Source: CAD feature listing. Evaluate the final solid. Frame: model axes, mm. A direction names the side the tool comes from. Give positions to 0.01 mm unless a question says otherwise; leave off trailing zeros. Order: outer loops, then holes, each group sorted by start corner. A loop starts at its lowest first (then second) coordinate and runs counter-clockwise, first axis right, second up.
```python
from build123d import *

# Parameters (mm, degrees)
SKETCH1_W           = 200
SKETCH1_H           = 200
BOSS_EXTRUDE2_DEPTH = 100
BOSS_EXTRUDE3_DEPTH = 10
CUT_EXTRUDE1_DEPTH  = 10
SKETCH4_W           = 120
SKETCH4_H           = 20
SKETCH4_W_2         = 20
SKETCH4_H_2         = 120
CUT_EXTRUDE2_DEPTH  = 229.910462845
SKETCH5_R           = 5
CUT_EXTRUDE3_DEPTH  = 314.687742827
SKETCH6_R           = 5
CUT_EXTRUDE4_DEPTH  = 288.054001888
SKETCH7_W           = 103.597474358
SKETCH7_H           = 100
CUT_EXTRUDE7_DEPTH  = 281.178514522
FILLET1_R           = 20


with BuildPart() as part:
    # Sketch1 → Boss-Extrude2 (new body)
    with BuildSketch(Plane(origin=(0, 0, 0), x_dir=(1, 0, 0), z_dir=(0, 1, 0))):
        Rectangle(SKETCH1_W, SKETCH1_H)
    extrude(amount=BOSS_EXTRUDE2_DEPTH)

    # Sketch2 → Boss-Extrude3 (add)
    with BuildSketch(Plane.ZY.offset(-100)):
        with BuildLine():
            Line((140, 10), (-140, 10))
            ThreePointArc((-140, 10), (-180, 50), (-140, 90))
            Line((-140, 90), (140, 90))
            ThreePointArc((140, 90), (180, 50), (140, 10))
        make_face()
    extrude(amount=BOSS_EXTRUDE3_DEPTH)

    # Sketch3 → Cut-Extrude1 (cut)
    with BuildSketch(Plane(origin=(0, 100, 0), x_dir=(1, 0, 0), z_dir=(0, 1, 0))):
        Polygon((8, 25), (8, 50), (94.602540378, 0), (8, -50), (8, -25), (-92, -25), (-92, 25), align=None)
    extrude(amount=-CUT_EXTRUDE1_DEPTH, mode=Mode.SUBTRACT)

    # Sketch4 → Cut-Extrude2 (cut, through all)
    with BuildSketch(Plane(origin=(0, 100, 0), x_dir=(1, 0, 0), z_dir=(0, 1, 0))):
        with Locations((20, 0)):
            Rectangle(SKETCH4_W, SKETCH4_H)
        with Locations((-70, 0)):
            Rectangle(SKETCH4_W_2, SKETCH4_H_2)
    extrude(amount=-CUT_EXTRUDE2_DEPTH, mode=Mode.SUBTRACT)

    # Sketch5 → Cut-Extrude3 (cut, through all)
    with BuildSketch(Plane.XY.offset(100)):
        with Locations((20.147207668, 50)):
            Circle(SKETCH5_R)
    extrude(amount=-CUT_EXTRUDE3_DEPTH, mode=Mode.SUBTRACT)

    # Sketch6 → Cut-Extrude4 (cut, through all)
    with BuildSketch(Plane.ZY.offset(100)):
        with Locations((0, 50)):
            Circle(SKETCH6_R)
    extrude(amount=-CUT_EXTRUDE4_DEPTH, mode=Mode.SUBTRACT)

    # Sketch7 → Cut-Extrude7 (cut, through all)
    with BuildSketch(Plane.ZY.offset(-90)):
        with Locations((-128.201262821, 50)):
            Rectangle(SKETCH7_W, SKETCH7_H)
        with Locations((128.201262821, 50)):
            Rectangle(SKETCH7_W, SKETCH7_H)
    extrude(amount=CUT_EXTRUDE7_DEPTH, mode=Mode.SUBTRACT)

    # Fillet1
    # the kernel refuses this fillet: 20 mm, written as the material it adds along each edge
    with BuildSketch(Plane(origin=(100, 10, -100), x_dir=(0, -1, 0), z_dir=(-1, 0, 0)), Plane(origin=(90, 10, 100), x_dir=(0, -1, 0), z_dir=(1, 0, 0))) as fillet1_piece_1:
        with BuildLine():
            CenterArc((20, -17.320508076), FILLET1_R, 120, 60)
            Line((0, -17.320508076), (-0.4, -17.320508076))
            Line((-0.4, -17.320508076), (-0.4, 0))
            Line((-0.4, 0), (0, 0.4))
            ThreePointArc((0, 0.4), (5, 0.4), (9.8, 0.346410162))
            Line((9.8, 0.346410162), (10, 0))
        make_face()
    extrude(amount=10)
    with BuildSketch(Plane(origin=(90, 90, -100), x_dir=(0, 0, -1), z_dir=(1, 0, 0)), Plane(origin=(100, 90, 100), x_dir=(0, 0, 1), z_dir=(-1, 0, 0))) as fillet1_piece_2:
        with BuildLine():
            CenterArc((17.320508076, 20), FILLET1_R, 210, 60)
            Line((0, 10), (-0.346410162, 9.8))
            ThreePointArc((-0.346410162, 9.8), (-0.4, 5), (-0.4, 0))
            Line((-0.4, 0), (0, -0.4))
            Line((0, -0.4), (17.320508076, -0.4))
            Line((17.320508076, -0.4), (17.320508076, 0))
        make_face()
    extrude(amount=10)


solid = part.part
```
1) Section query B-B, the plane x = 3. Return the cut outline in (y, z).
Report:
outline: (0, -76.4) - (100, -76.4) - (100, -25) - (90, -25) - (90, -10) - (0, -10) - close; (0, 10) - (90, 10) - (90, 25) - (100, 25) - (100, 76.4) - (0, 76.4) - close
2) Material intervals for L1, parallel to X at y = 36.5, z = 7; L2, parallel to Z at x = -90.5, y = 94.5; L3, parallel to Y at x = 95, z = 0, sorted ascending.
Report:
L1: x = -100 to -80, -60 to -40, 80 to 100
L2: z = -76.4 to -25, 25 to 76.4
L3: y = 0 to 45, 55 to 100
3) Section query A-A, the plane z = -56. Return the cut outline in (x, y), and give its area (3 significant figures).
Report:
outline: (-100, 0) - (-80, 0) - (-80, 100) - (-100, 100) - close; (-60, 0) - (100, 0) - (100, 100) - (-60, 100) - close; hole circle Ø10 at (20.15, 50)
area: 17,900 mm2
4) Reachability of faces 4 (the flat face through (95, 90, -129)), 5 (the flat face through (19, 40, -10)), 6 (the flat face through (-26, 95, 25)) from +Z, -Z, +X, -X, +Y, -Y: full face, straight path, thin tool, end or side. Return the list, or none.
Report:
face 4: -Z, +X, -X, +Y
face 5: +Y, -Y
face 6: +Y
5) Pin query (flat end, axial travel): pin 1 (8 mm diameter, centred on x = 94.5, z = -132.5, fed in from -Y); pin 2 (6 mm diameter, centred on x = 20.15, y = 50, fed in from -Z); pin 3 (12 mm diameter, centred on x = 34, y = 17.5, fed in from +Z); pin 4 (22 mm diameter, centred on x = -69, y = 61.5, fed in from -Z). Return the tip coordinate at first contact, or that it passes through.
Report:
pin 1: stops at y = 10
pin 2: passes through
pin 3: stops at z = 76.4
pin 4: stops at z = -76.4
6) Draft query along Z for faces 1 (the flat face through (-100, 38, 1)), 2 (the flat face through (8, 95, -37)), 3 (the cylindrical face through (94.93, 92.753, -107.194)). Return one class per face: +Z half, -Z half, draft (parallel to the pull), parting line (faces both ways), or undercut.
Report:
face 1: draft
face 2: undercut
face 3: -Z half
7) Section query C-C, the plane y = 66.5. Return the cut outline in (x, z), and give its area (3 significant figures).
Report:
outline: (-100, -76.4) - (90, -76.4) - (90, -176.44) - (100, -176.44) - (100, 176.44) - (90, 176.44) - (90, 76.4) - (-100, 76.4) - close; hole (-80, -60) - (-60, -60) - (-60, 60) - (-80, 60) - close; hole (-40, -10) - (80, -10) - (80, 10) - (-40, 10) - close
area: 27,800 mm2
8) Section query D-D, the plane y = 50. Count the separate pieces of the cut face and the enclosed holes in it, and give its area (3 significant figures).
Report:
separate pieces: 4
enclosed holes: 0
area: 25,900 mm2
